from build123d import *

# Parameters (mm, degrees)
F0_W     = 127
F0_H     = 508
F0_W_2   = 19.558
F0_H_2   = 83.82
F0_R     = 12.7
F1_DEPTH = 18.415


with BuildPart() as f1:
    # F0 (on Top) → F1 (new body)
    with BuildSketch(Plane.XY):
        with BuildLine():
            ThreePointArc((5.986409, 152.4), (50.623336, 44.636927), (158.386409, 0))
            Line((158.386409, 0), (615.586409, 0))
            ThreePointArc((615.586409, 0), (723.349482, 44.636927), (767.986409, 152.4))
            Line((767.986409, 152.4), (767.986409, 1168.4))
            Line((767.986409, 1168.4), (577.486409, 1803.4))
            Line((577.486409, 1803.4), (577.486409, 2311.4))
            Line((577.486409, 2311.4), (196.486409, 2311.4))
            Line((196.486409, 2311.4), (196.486409, 1803.4))
            Line((196.486409, 1803.4), (5.986409, 1168.4))
            Line((5.986409, 1168.4), (5.986409, 152.4))
        make_face()
        with Locations((386.986409, 355.6)):
            Rectangle(F0_W, F0_H, mode=Mode.SUBTRACT)
        with Locations((66.565409, 610.87)):
            Rectangle(F0_W_2, F0_H_2, mode=Mode.SUBTRACT)
        with Locations((66.565409, 745.49)):
            Rectangle(F0_W_2, F0_H_2, mode=Mode.SUBTRACT)
        with Locations((707.407409, 610.87)):
            Rectangle(F0_W_2, F0_H_2, mode=Mode.SUBTRACT)
        with Locations((707.407409, 745.49)):
            Rectangle(F0_W_2, F0_H_2, mode=Mode.SUBTRACT)
        with Locations((386.986409, 2184.4)):
            Circle(F0_R, mode=Mode.SUBTRACT)
    extrude(amount=F1_DEPTH)


solid = f1.part
Part model, mm, in its own coordinate system. Give positions to 0.01 mm unless a question says otherwise; leave off trailing zeros. Loops run counter-clockwise (first coordinate to the right, second up) from the corner with the lowest first, then second, coordinate; pieces in that order, holes last. Notation, with made-up numbers: (84.5, 37) -> (117.5, 37) arc R9 cw to (117.5, 42) -> close; hole circle Ø10 at (-20.75, -6.75). An arc over 180 degrees is marked (long way). Write each question's results on one line, items separated by ' | '. Start each with the question number.
Q1. Pin check, flat tips, straight feed: P1, Ø5.5, axis at x = 707, z = 8, coming from the -Y side; P2, Ø1, axis at y = 1708.5, z = 15.5, coming from the +X side. Stop position of each tip, or through.
Q2. Pull direction Y, two halves, no side cores. Call faces 1 (the face through (49.445, 45.828, 9.079)), 2 (the face through (382, 1172, 0)), 3 (the face through (102.57, 1490.34, 9.08)): +Y half, -Y half, draft (parallel to the pull), parting line (faces both ways), or undercut.
Q3. Band-saw the part on B-B on x = 96.5. List the corners of the cut face in (y, z) (3 decimals), plus the area to 3 significant figures.
Q4. Band-saw the part on A-A on z = 8. Count the separate pieces of the cut face and the enclosed holes in it, plus the area to 3 significant figures.
Q5. Wall check: L1, parallel to X at y = 605, z = 4.5; L2, parallel to X at y = 2184.4, z = 4.75; L3, parallel to X at y = 243, z = 4.25. Give the ranges that are in metal, low to high.
Results are:
1) P1: stops at y = 28.45 | P2: stops at x = 606.11
2) face 1: -Y half | face 2: draft | face 3: +Y half
3) outline: (13.131, 0) -> (1470.112, 0) -> (1470.112, 18.415) -> (13.131, 18.415) -> close | area: 26,800 mm²
4) separate pieces: 1 | enclosed holes: 6 | area: 1,370,000 mm²
5) L1: x = 5.99 to 56.79, 76.34 to 323.49, 450.49 to 697.63, 717.19 to 767.99 | L2: x = 196.49 to 374.29, 399.69 to 577.49 | L3: x = 5.99 to 323.49, 450.49 to 767.99
